```python
from build123d import *

# Parameters (mm, degrees)
SKETCH_1_W          = 29.6
SKETCH_1_H          = 28.73
EXTRUDE_1_DEPTH     = 47.23
SKETCH_2_W          = 29.6
SKETCH_2_H          = 24.73
CUT_EXTRUDE_1_DEPTH = 45.23
SKETCH_3_W          = 8
SKETCH_3_H          = 28.73
EXTRUDE_2_DEPTH     = 2
SKETCH_4_W          = 29.6
SKETCH_4_H          = 6
EXTRUDE_3_DEPTH     = 2
SKETCH_5_R          = 1.5
CUT_EXTRUDE_2_DEPTH = 53.37104281


with BuildPart() as part:
    # 草图1 → 凸台-拉伸1 (new body)
    with BuildSketch(Plane.XY):
        Rectangle(SKETCH_1_W, SKETCH_1_H)
    extrude(amount=EXTRUDE_1_DEPTH)

    # 草图2 → 切除-拉伸1 (cut)
    with BuildSketch(Plane.XY.offset(47.23)):
        Rectangle(SKETCH_2_W, SKETCH_2_H)
    extrude(amount=-CUT_EXTRUDE_1_DEPTH, mode=Mode.SUBTRACT)

    # 草图3 → 凸台-拉伸2 (add)
    with BuildSketch(Plane.ZY.offset(14.8)):
        with Locations((4, 0)):
            Rectangle(SKETCH_3_W, SKETCH_3_H)
    extrude(amount=EXTRUDE_2_DEPTH)

    # 草图4 → 凸台-拉伸3 (add)
    with BuildSketch(Plane.XY.offset(47.23)):
        with Locations((0, 17.365)):
            Rectangle(SKETCH_4_W, SKETCH_4_H)
    extrude_3 = extrude(amount=-EXTRUDE_3_DEPTH)

    # 草图5 → 切除-拉伸2 (cut, through all)
    with BuildSketch(Plane(origin=(0, 0, 45.23), x_dir=(-1, 0, 0), z_dir=(0, 0, -1))):
        with Locations((-9.8, 17.365)):
            Circle(SKETCH_5_R)
        with Locations((9.8, 17.365)):
            Circle(SKETCH_5_R)
    cut_extrude_2 = extrude(amount=-CUT_EXTRUDE_2_DEPTH, mode=Mode.SUBTRACT)

    # 镜向2: 凸台-拉伸3, 切除-拉伸2 across plane
    add(extrude_3.mirror(Plane.ZX))
    add(cut_extrude_2.mirror(Plane.ZX), mode=Mode.SUBTRACT)


solid = part.part
```
Can you work these out from the model? Positions are in its coordinate system, mm. A direction names the side the tool comes from. Coordinates: 2 decimals unless noted, no trailing zeros. Loops run counter-clockwise (first coordinate to the right, second up) from the corner with the lowest first, then second, coordinate; pieces in that order, holes last. Notation, with made-up numbers: (-38, -17) -> (-15, -17) arc R23 ccw to (-15, 22) -> close; hole circle Ø11 at (35, -1). An arc over 180 degrees is marked (long way). Put each result on its own line as item: value. Start each with the question number.
Q1. I want a section at B-B (x = -9.8). Write out the boundary of the cut face in (y, z) (3 decimals).
Q2. Thinking about a two-plate mould opening in Y: for faces 4 (the face through (8.994, -18.63, 46.216)), 5 (the face through (0, 12.365, 25)), 6 (the face through (0, -17, 45.23)), 7 (the face through (-1, 14.365, 22)), which applies, pulls with the +Y half, pulls with the -Y half, needs draft (parallel to the pull), parting line crosses it, or undercut?
Q3. I want a section at A-A (z = 41). Write out the boundary of the cut face in (x, y) (3 decimals), plus the area to 3 significant figures.
Q4. I want a section at C-C (y = 4). Write out the boundary of the cut face in (x, z).
Q5. If I drill on line 1 (Y direction, x = 13.5, z = 38) (3 decimals); line 2 (Y direction, x = -9, z = 46) (3 decimals); line 3 (Z direction, x = 3.5, y = -2), over which ranges is the centre line in solid material (lowest first)? Write a range as [from, to].
Q6. I want a section at D-D (x = 1). Write out the boundary of the cut face in (y, z) (3 decimals).
Q7. For faces 1 (the face through (0, 0, 2)), 2 (the face through (0, 17, 45.23)), 3 (the face through (-16, 0, 8)), which set-ups out of +Z, -Z, +X, -X, +Y, -Y let a thin tool reach every point of the face, with its end or its side?
Q8. I'm going to push flat-ended pins straight in: P1, Ø2.5, axis at x = -9.8, y = 17.365, coming from the -Z side; P2, Ø1, axis at y = 13, z = 23.5, coming from the -X side; P3, Ø12, axis at x = -11, z = 17, coming from the -Y side (3 decimals); P4, Ø5, axis at x = 0, y = -18.5, coming from the -Z side. Where does each tip first touch, or does it pass through?
Taken from the geometry:
1. outline: (-20.365, 45.23) -> (-18.865, 45.23) -> (-18.865, 47.23) -> (-20.365, 47.23) -> close; (-15.865, 45.23) -> (-14.365, 45.23) -> (-14.365, 0) -> (14.365, 0) -> (14.365, 45.23) -> (15.865, 45.23) -> (15.865, 47.23) -> (12.365, 47.23) -> (12.365, 2) -> (-12.365, 2) -> (-12.365, 47.23) -> (-15.865, 47.23) -> close; (18.865, 45.23) -> (20.365, 45.23) -> (20.365, 47.23) -> (18.865, 47.23) -> close
2. face 4: undercut
2. face 5: undercut
2. face 6: needs draft
2. face 7: pulls with the +Y half
3. outline: (-14.8, -14.365) -> (14.8, -14.365) -> (14.8, -12.365) -> (-14.8, -12.365) -> close; (-14.8, 12.365) -> (14.8, 12.365) -> (14.8, 14.365) -> (-14.8, 14.365) -> close
3. area: 118 mm2
4. outline: (-16.8, 0) -> (14.8, 0) -> (14.8, 2) -> (-14.8, 2) -> (-14.8, 8) -> (-16.8, 8) -> close
5. line 1: y = [-14.365, -12.365], [12.365, 14.365]
5. line 2: y = [-20.365, -18.634], [-16.096, -12.365], [12.365, 16.096], [18.634, 20.365]
5. line 3: z = [0, 2]
6. outline: (-20.365, 45.23) -> (-14.365, 45.23) -> (-14.365, 0) -> (14.365, 0) -> (14.365, 45.23) -> (20.365, 45.23) -> (20.365, 47.23) -> (12.365, 47.23) -> (12.365, 2) -> (-12.365, 2) -> (-12.365, 47.23) -> (-20.365, 47.23) -> close
7. face 1: +Z, +X
7. face 2: -Z, +X, -X, +Y
7. face 3: +Z, -X, +Y, -Y
8. P1: passes through
8. P2: stops at x = -14.8
8. P3: stops at y = -14.365
8. P4: stops at z = 45.23
